For this review, take the finished solid that the model builds, in its own axes (mm). A direction names the side the tool comes from. Round coordinates to 2 decimals unless told otherwise and drop trailing zeros. Order: outer loops, then holes, each group sorted by start corner. A loop starts at its lowest first (then second) coordinate and runs counter-clockwise, first axis right, second up. Notation, with made-up numbers: (-9, 3) - (12, 3) arc R18 ccw to (12, 17) - close; hole circle Ø4 at (85, 21). An arc over 180 degrees is marked (long way). One line per item, written item: value.
Autodesk Inventor part; units mm, degrees
ref_plane "Work Plane1" through (-7.3684, -20.6375, 113.4742) normal (0.9769, 0, -0.2136969) x (-0.2136969, 0, -0.9769)
ref_plane "YZ Plane" through (0, 0, 0) normal (1, 0, 0) x (0, 1, 0)
ref_plane "XZ Plane" through (0, 0, 0) normal (0, 1, 0) x (-1, 0, 0)
sketch "Sketch1" plane through (0, 0, 0) normal (0, 1, 0) x (-1, 0, 0)
  line L0 (43.0137, 64.3915) -> (32.1817, 14.8739)
  line L1 (-10.5502, -12.5966) -> (-8.8333, -15.2673)
  line L2 (-8.8333, -15.2673) -> (35.0028, 12.913)
  line L3 (35.0028, 12.913) -> (46.1153, 63.713)
  line L4 (46.1153, 63.713) -> (43.0137, 64.3915)
  line L5 (-10.5502, -12.5966) -> (-10.5502, 12.913)
  line L6 (-10.5502, -12.5966) -> (32.1817, 14.8739)
  line L7 (46.1153, 63.713) -> (74.6903, 63.713)
  line L8 (74.6903, 63.713) -> (74.6903, 66.888)
  line L9 (74.6903, 66.888) -> (43.5598, 66.888)
  line L10 (43.0137, 64.3915) -> (43.5598, 66.888)
  point P0 (0, 0)
  dimension "d0" = 3.175
  dimension "d1" = 3.175
  dimension "d3" = 50.8
  dimension "d4" = 57.265
  dimension "d5" = 50.8
  dimension "d6" = 11.1125
  dimension "d7" = 28.575
  dimension "d8" = 3.175
extrude "Extrusion1" add sketch "Sketch1" along normal blind 28.575
sketch "Sketch2" plane through (-74.6903, 0, 66.888) normal (0, 0, 1) x (1, 0, 0)
  line L0 (28.575, 0) -> (0, 0)
  line L1 (0, 0) -> (0, 28.575)
  line L2 (28.575, 28.575) -> (0, 28.575)
  line L3 (28.575, 0) -> (28.575, 28.575)
  line L4 (28.575, 28.575) -> (0, 28.575)
  line L5 (0, 0) -> (0, 28.575)
  circle A0 centre (14.2875, 14.2875) radius 11.1125
  point P0 (74.6903, 0)
  point P1 (14.2875, 28.575)
  point P2 (0, 14.2875)
  dimension "d11" = 22.225
extrude "Extrusion2" cut sketch "Sketch2" against normal blind 28.575 contours A0
sketch "Sketch3" plane through (10.5502, 0, -12.5966) normal (0.5407576, 0, 0.8411785) x (0.8411785, 0, -0.5407576)
  line L0 (-50.8, 0) -> (-50.8, 28.575)
  line L1 (-50.8, 7.9375) -> (0, 7.9375)
  line L2 (0, 7.9375) -> (0, -20.6375)
  line L3 (0, -20.6375) -> (-50.8, -20.6375)
  line L4 (-50.8, -20.6375) -> (-50.8, 7.9375)
  line L5 (-50.8, 28.575) -> (0, 28.575)
  point P0 (-15.6863, 0)
  dimension "d14" = 50.8
  dimension "d15" = 28.575
  dimension "d16" = 20.6375
sketch "Sketch4" plane through (-32.1817, 0, 14.8739) normal (0.9769, 0, 0.2136969) x (0.2136969, 0, -0.9769)
  line L0 (-53.2441, 0) -> (-53.2441, 28.575)
  line L1 (-53.2441, 28.575) -> (0, 7.9375)
  line L2 (0, 0) -> (0, 28.575)
  line L3 (0, 7.9375) -> (0, -20.6375)
  line L4 (0, -20.6375) -> (-53.2441, 0)
  line L5 (-53.2441, 28.575) -> (-53.2441, 0)
  point P0 (21.4074, 0)
  dimension "d17" = 20.6375
  dimension "d18" = 28.575
sketch "Sketch5" plane through (-32.1817, 0, 14.8739) normal (0.9769, 0, 0.2136969) x (0.2136969, 0, -0.9769)
  line L0 (-53.2441, 41.9678) -> (42.8737, 41.9678)
  line L1 (42.8737, 41.9678) -> (42.8737, -28.4609)
  line L2 (42.8737, -28.4609) -> (-53.2441, -28.4609)
  line L3 (-53.2441, -28.4609) -> (-53.2441, 41.9678)
  point P0 (21.4074, 0)
extrude "Extrusion3" cut sketch "Sketch5" along normal blind 50.8 and the other way blind 3.175
extrude "Extrusion4" add sketch "Sketch4" against normal blind 3.175
extrude "Extrusion5" add sketch "Sketch3" against normal blind 3.175
sketch "Sketch6" plane through (8.8333, 0, -15.2673) normal (-0.5407576, 0, -0.8411785) x (-0.8411785, 0, 0.5407576)
  line L0 (50.8, 7.9375) -> (0, 7.9375)
  line L1 (50.8, 7.9375) -> (63.8738, 7.9375)
  line L2 (63.8738, 7.9375) -> (63.8738, -20.6375)
  line L3 (63.8738, -20.6375) -> (50.8, -20.6375)
  line L4 (50.8, -20.6375) -> (50.8, 7.9375)
  point P0 (15.6863, 0)
extrude "Extrusion6" add sketch "Sketch6" against normal blind 3.175
sketch "Sketch7" plane through (-35.2833, 0, 14.1954) normal (-0.9769, 0, -0.2136969) x (-0.2136969, 0, 0.9769)
  line L0 (50.6885, 27.5845) -> (0, 7.9375)
  line L1 (3.1832, -19.4037) -> (53.2441, 0)
  line L2 (0, 7.9375) -> (3.1832, 7.9375)
  line L3 (0, 7.9375) -> (-56.9759, -14.1465)
  line L4 (-56.9759, -14.1465) -> (-50.1301, -40.068)
  line L5 (53.2441, 0) -> (0, -20.6375)
  line L6 (-50.1301, -40.068) -> (0, -20.6375)
  line L7 (0, 7.9375) -> (-35.9676, 7.9375)
  line L8 (0, 7.9375) -> (0, -20.6375)
  line L9 (11.5155, 12.4009) -> (21.1446, -12.4418)
  line L10 (-34.1585, 31.8696) -> (27.6424, 31.8696)
  line L11 (27.6424, 31.8696) -> (27.6424, -37.0154)
  line L12 (27.6424, -37.0154) -> (-34.1585, -37.0154)
  line L13 (-34.1585, -37.0154) -> (-34.1585, 31.8696)
  point P0 (-21.4074, 0)
extrude "Extrusion7" cut sketch "Sketch7" along normal blind 25.4 contours L9 L1 L5 L8 L0 | L0 L7 L13 L10 L11 | L0 L11 L1 L9 | L8 L6 L13 L3 | L3 L13 L7 | L1 L11 L12 L13 L6 L5
mirror "Mirror1" about plane through (-74.6903, 0, 66.888) normal (0, 0, 1)
sketch "Sketch8" plane through (0, 28.575, 0) normal (0, 1, 0) x (1, 0, 0)
  line L0 (-74.6903, -63.713) -> (-74.6903, -70.063)
  line L1 (-74.6903, -66.888) -> (15.7413, -66.888)
  line L2 (15.7413, -66.888) -> (15.7413, 23.0839)
  line L3 (15.7413, 23.0839) -> (-74.6903, 23.0839)
  line L4 (-74.6903, 23.0839) -> (-74.6903, -66.888)
  point P0 (0, 0)
extrude "Extrusion8" cut sketch "Sketch8" against normal blind 49.2125
ref_plane "Work Plane1" through (-7.3684, -20.6375, 113.4742) normal (0.9769, 0, -0.2136969) x (-0.2136969, 0, -0.9769)
sketch "Sketch10" plane through (0, 28.575, 0) normal (0, 1, 0) x (1, 0, 0)
  line L0 (-1.9264, -138.3519) -> (-5.0281, -139.0304)
  line L1 (-1.9264, -138.3519) -> (-13.3045, -86.3378)
  line L2 (-46.6614, -54.5282) -> (-5.0281, -54.5282)
  line L3 (-5.0281, -54.5282) -> (-5.0281, -144.0467)
  line L4 (-5.0281, -144.0467) -> (-46.6614, -144.0467)
  line L5 (-46.6614, -144.0467) -> (-46.6614, -54.5282)
  point P0 (0, 0)
  dimension "d35" = 3.175
extrude "Extrusion9" cut sketch "Sketch10" against normal blind 57.15 contours L3 L4 L5 L2
sketch "Sketch11" plane through (0, 28.575, 0) normal (0, 1, 0) x (1, 0, 0)
  line L0 (-74.6903, -66.888) -> (-46.6614, -66.888)
  line L1 (-46.6614, -66.888) -> (-46.1153, -66.888)
  line L2 (-46.1153, -66.888) -> (-46.1153, -70.063)
  line L3 (-46.1153, -70.063) -> (-46.6614, -70.063)
  line L4 (-46.6614, -70.063) -> (-46.6614, -66.888)
  line L5 (-74.6903, -66.888) -> (-74.6903, -70.063)
  point P0 (0, 0)
  dimension "d38" = 28.575
extrude "Extrusion10" add sketch "Sketch11" against normal up to surface (28.575 mm away)
sketch "Sketch12" plane through (-74.6903, 0, 66.888) normal (0, 0, -1) x (-1, 0, 0)
  line L0 (0, 0) -> (-28.575, 0)
  line L1 (0, 28.575) -> (0, 0)
  line L2 (-28.575, 28.575) -> (0, 28.575)
  line L3 (-28.575, 28.575) -> (-28.575, 0)
  circle A0 centre (-14.2875, 14.2875) radius 11.1125
  point P0 (-74.6903, 0)
extrude "Extrusion11" add sketch "Sketch12" along normal blind 6.35
sketch "Sketch13" plane through (-74.6903, 0, 70.063) normal (0, 0, 1) x (1, 0, 0)
  line L0 (28.575, 28.575) -> (0, 28.575)
  line L1 (0, 0) -> (0, 28.575)
  line L2 (28.575, 0) -> (0, 0)
  line L3 (28.575, 28.575) -> (28.575, 0)
  circle A0 centre (14.2875, 14.2875) radius 11.1125
  point P0 (74.6903, 0)
extrude "Extrusion12" cut sketch "Sketch13" against normal blind 6.35
sketch "Sketch14" plane through (-7.3684, -20.6375, 113.4742) normal (0.9769, 0, -0.2136969) x (-0.2136969, 0, -0.9769)
  line L0 (-22.8553, 28.575) -> (-26.5426, 28.575)
  line L1 (59.9935, 49.2125) -> (59.9935, 20.6375)
  line L2 (-22.8553, 28.575) -> (59.9935, 49.2125)
  line L3 (59.9935, 20.6375) -> (66.0999, 20.6375)
  line L4 (59.9935, 49.2125) -> (59.9935, 20.6375)
  line L5 (-22.8553, 0) -> (-22.8553, 28.575)
  line L6 (59.9935, 20.6375) -> (-22.8553, 0)
  line L7 (-22.8553, 0) -> (-22.8553, 28.575)
  point P0 (109.2784, 20.6375)
extrude "Extrusion13" add sketch "Sketch14" against normal blind 3.175
sketch "Sketch16" plane through (-46.1153, 0, 60.538) normal (1, 0, 0) x (0, 0, -1)
  line L0 (-3.175, 28.575) -> (-3.175, 0)
  line L1 (-3.175, 0) -> (0, 0)
  line L2 (0, 28.575) -> (0, 0)
  line L3 (-3.175, 28.575) -> (0, 28.575)
  point P0 (60.538, 0)
extrude "Extrusion14" add sketch "Sketch16" along normal blind 33.3375
sketch "Sketch17" plane through (-7.3684, -20.6375, 113.4742) normal (0.9769, 0, -0.2136969) x (-0.2136969, 0, -0.9769)
  line L0 (39.8727, 61.7245) -> (70.5453, 61.7245)
  line L1 (70.5453, 61.7245) -> (70.5453, 3.8032)
  line L2 (70.5453, 3.8032) -> (39.8727, 3.8032)
  line L3 (39.8727, 3.8032) -> (39.8727, 61.7245)
  point P0 (109.2784, 20.6375)
extrude "Extrusion15" cut sketch "Sketch17" along normal blind 33.3375
sketch "Sketch18" plane through (0, 28.575, 0) normal (0, 1, 0) x (1, 0, 0)
  line L0 (-74.6903, -60.538) -> (-18.9482, -60.538)
  line L1 (-26.1324, -60.538) -> (-14.0387, -60.538)
  line L2 (-14.0387, -60.538) -> (-14.0387, -48.514)
  line L3 (-14.0387, -48.514) -> (-26.1324, -48.514)
  line L4 (-26.1324, -48.514) -> (-26.1324, -60.538)
  point P0 (0, 0)
extrude "Extrusion16" cut sketch "Sketch18" against normal blind 33.3375
sketch "Sketch19" plane through (0, 28.575, 0) normal (0, 1, 0) x (1, 0, 0)
  line L0 (-21.5038, -63.713) -> (-74.6903, -63.713)
  line L1 (-28.5092, -63.713) -> (0.9764, -63.713)
  line L2 (0.9764, -63.713) -> (0.9764, -136.358)
  line L3 (0.9764, -136.358) -> (-28.5092, -136.358)
  line L4 (-28.5092, -136.358) -> (-28.5092, -63.713)
  point P0 (0, 0)
extrude "Extrusion17" cut sketch "Sketch19" against normal blind 82.55
sketch "Sketch20" plane through (0, 28.575, 0) normal (0, 1, 0) x (1, 0, 0)
  line L0 (-74.6903, -60.538) -> (-22.1983, -60.538)
  line L1 (-21.5038, -63.713) -> (-74.6903, -63.713)
  line L2 (-74.6903, -60.538) -> (-23.8903, -60.538)
  line L3 (-23.8903, -60.538) -> (-23.8903, -63.713)
  line L4 (-23.8903, -63.713) -> (-74.6903, -63.713)
  line L5 (-74.6903, -63.713) -> (-74.6903, -60.538)
  line L6 (-23.8903, -55.4967) -> (-9.2163, -55.4967)
  line L7 (-9.2163, -55.4967) -> (-9.2163, -75.9107)
  line L8 (-9.2163, -75.9107) -> (-23.8903, -75.9107)
  line L9 (-23.8903, -75.9107) -> (-23.8903, -55.4967)
  point P0 (0, 0)
  dimension "d55" = 50.8
extrude "Extrusion18" cut sketch "Sketch20" against normal blind 82.55 contours L9 L6 L7 L8 L3
sketch "Sketch21" plane through (-5.0281, 7.9375, 140.1325) normal (0, 1, 0) x (1, 0, 0)
  line L0 (15.5783, -6.2401) -> (13.8614, -8.9109)
  line L1 (13.8614, -8.9109) -> (15.5783, -6.2401)
  line L2 (15.5783, -6.2401) -> (-5.7877, 7.4951)
  line L3 (-5.7877, 7.4951) -> (-7.5046, 4.8244)
  line L4 (-7.5046, 4.8244) -> (13.8614, -8.9109)
  point P0 (5.0281, 140.1325)
  dimension "d58" = 25.4
extrude "Extrusion19" add sketch "Sketch21" against normal blind 28.575
sketch "Sketch22" plane through (-5.6127, 7.9375, 136.358) normal (0, 1, 0) x (1, 0, 0)
  line L0 (-48.2657, 34.2615) -> (88.3828, 30.5881)
  line L1 (88.3828, 30.5881) -> (85.9509, -59.8767)
  line L2 (85.9509, -59.8767) -> (-50.6975, -56.2034)
  line L3 (-50.6975, -56.2034) -> (-48.2657, 34.2615)
  point P0 (5.6127, 136.358)
extrude "Extrusion20" cut sketch "Sketch22" along normal blind 28.575
sketch "Sketch23" plane through (-74.6903, 0, 63.713) normal (0, 0, 1) x (1, 0, 0)
  line L0 (0, 28.575) -> (50.8, 28.575)
  line L1 (50.8, 0) -> (0, 0)
  line L2 (50.8, 28.575) -> (47.625, 28.575)
  line L3 (47.625, 28.575) -> (47.625, 0)
  line L4 (47.625, 0) -> (50.8, 0)
  line L5 (50.8, 0) -> (50.8, 28.575)
  point P0 (74.6903, 0)
  dimension "d63" = 3.175
loft "Loft1" add profiles "Sketch23" section 2 edges at (-11.6742, 7.9375, 133.9728) (-10.8157, -6.35, 132.6374) (-11.6742, -20.6375, 133.9728) (-12.5326, -6.35, 135.3081)
sketch "Sketch26" plane through (-74.6903, 0, 60.538) normal (0, 0, -1) x (-1, 0, 0)
  line L0 (-50.8, 0) -> (-50.8, 28.575)
  ellipse E0 centre (-50.8, 0) end of major axis (-31.75, 0) minor radius 12.7
  point P0 (-74.6903, 0)
  dimension "d71" = 12.7
  dimension "d72" = 19.05
extrude "Extrusion22" cut sketch "Sketch26" against normal blind 12.7
properties part number "Spinner to Top Other Side"
Item 1: Take a section at B-B (y = 9). Count the separate pieces of the cut face and the enclosed holes in it, plus the area to 3 significant figures.
Returned:
separate pieces: 3
enclosed holes: 0
area: 209 mm^2
Item 2: Take a section at A-A (x = -60). Write out the cut boundary in (y, z) (3 decimals).
Returned:
outline: (0, 60.538) - (3.182, 60.538) - (3.182, 63.713) - (0, 63.713) - close; (25.393, 60.538) - (28.575, 60.538) - (28.575, 63.713) - (25.393, 63.713) - close
Item 3: Wall thickness on line 1 (Z direction, x = -48, y = 1.5); line 2 (Z direction, x = -7, y = 0); line 3 (X direction, y = 7, z = 121): over which ranges is each line inside the solid? List them lowest first.
Returned:
line 1: 60.54 to 63.71
line 2: 135.09 to 138.86
line 3: -15.44 to -13.02
Item 4: Machinability: for faces 1 (the flat face through (-51, 21, 63.713)), 2 (the flat face through (-49.6, 17.7, 60.538)), which of the approach directions +Z, -Z, +X, -X, +Y, -Y give a long, thin tool a straight path to every point of the face, cutting with its end or side? Answer none if there is none.
Returned:
face 1: +Z, -X, +Y, -Y
face 2: -Z, +X, -X, +Y, -Y
Item 5: For P1, Ø3, axis at x = -51, y = 13, coming from the -Z side; P2, Ø4, axis at y = -1, z = 129, coming from the -X side; P3, Ø4, axis at x = -42, y = 13.5, coming from the +Z side; P4, Ø3.5, axis at x = -24, y = 5, coming from the -Z side, all flat-tipped, find the tip position at first contact; note any pin that passes through.
Returned:
P1: through
P2: x = -14.22
P3: z = 63.71
P4: z = 73.24
Item 6: The part is to be moulded in two halves that separate along X. For faces 3 (the flat face through (-50, 28.575, 62)), 4 (the cylindrical face through (-70.67, 18.54, 62.15)), 5 (the flat face through (-23.89, 21, 62)), say which applies: +X half, -X half, draft (parallel to the pull), parting line (faces both ways), or undercut.
Returned:
face 3: draft
face 4: undercut
face 5: +X half
Item 7: Take a section at C-C (z = 143.5). Write out the cut boundary in (x, y).
Returned:
outline: (0.21, -20.64) - (6.08, -20.64) - (6.08, 7.94) - (0.21, 7.94) - close
